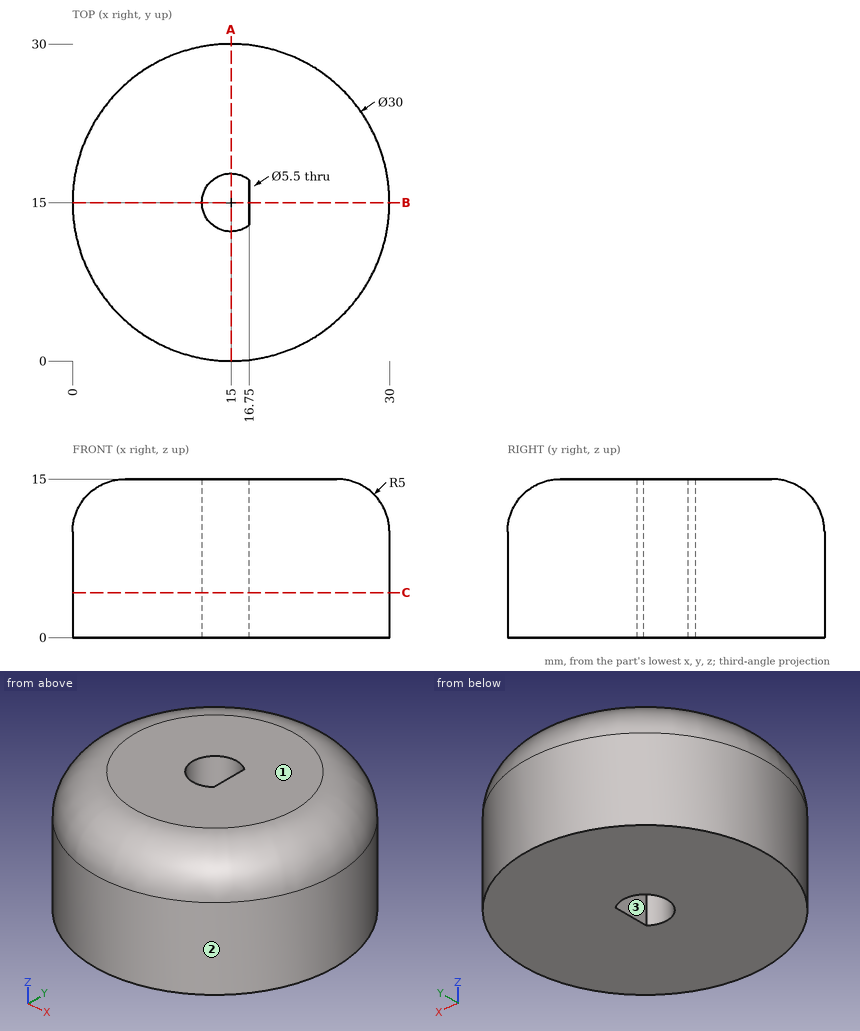
Here's the drawing with two shaded views (mm, measured from the low corner). I have some questions. Give positions to 0.01 mm unless a question says otherwise; leave off trailing zeros. Write each loop counter-clockwise with the first axis right and the second up, starting at its lowest first coordinate (ties: lowest second). Pieces come first, ordered by that corner, then holes. Notation, with made-up numbers: (73.25, 51) - (117.25, 51) arc R23 cw to (117.25, 79) - close; hole circle Ø7 at (10.5, 4.25). An arc over 180 degrees is marked (long way). One line per item, written item: value. Start each with the question number.
Item 1: Imagine slicing it at C-C, the plane z = 4.25. List the corners of the cut face in (x, y) for me.
Item 2: I'm going to push flat-ended pins straight in: pin 1 (4 mm diameter, centred on x = 20, z = 1.5, fed in from -Y); pin 2 (8 mm diameter, centred on x = 25, z = 10, fed in from -Y); pin 3 (1.5 mm diameter, centred on y = 20.5, z = 5, fed in from +X). Where does each tip first touch, or does it pass through?
Item 3: If we mould it in two halves opening along X, with no side actions, what happens to the marked faces 1, 2 and 3? For each: +X half, -X half, draft (parallel to the pull), parting line (faces both ways), or undercut.
Item 4: Please list where these lines run through material, in increasing order: line 1 (Y direction, x = 15, z = 7); line 2 (Y direction, x = 12.5, z = 6). Write a range as from..to.
Item 5: Imagine slicing it at A-A, the plane x = 15. List the corners of the cut face in (y, z) for me, and give its area (3 significant figures).
Item 6: Imagine slicing it at B-B, the plane y = 15. List the corners of the cut face in (x, z) for me.
Geometry says:
1. outline: circle Ø30 at (15, 15); hole (16.75, 12.88) - (16.75, 17.12) arc R2.75 ccw (long way) to start
2. pin 1: y = 0.3
2. pin 2: y = 1.25
2. pin 3: x = 29.23
3. face 1: draft
3. face 2: parting line
3. face 3: undercut
4. line 1: 0..12.25, 17.75..30
4. line 2: 0.21..13.85, 16.15..29.79
5. outline: (0, 0) - (12.25, 0) - (12.25, 15) - (5, 15) arc R5 ccw to (0, 10) - close; (17.75, 0) - (30, 0) - (30, 10) arc R5 ccw to (25, 15) - (17.75, 15) - close
5. area: 357 mm^2
6. outline: (0, 0) - (12.25, 0) - (12.25, 15) - (5, 15) arc R5 ccw to (0, 10) - close; (16.75, 0) - (30, 0) - (30, 10) arc R5 ccw to (25, 15) - (16.75, 15) - close
